```python
from build123d import *

# Parameters (mm, degrees)
F1_DEPTH = 160
F3_DEPTH = 120
F5_DEPTH = 180
F6_R     = 6.35
F7_R     = 6.35


with BuildPart() as f1:
    # F0 (on Front) → F1 (new body)
    with BuildSketch(Plane.XZ):
        with BuildLine():
            Line((140.422905, 79.857803), (-26.877095, 79.857803))
            ThreePointArc((-26.877095, 79.857803), (-31.367223, 77.997931), (-33.227095, 73.507803))
            Line((-33.227095, 73.507803), (-33.227095, -33.792197))
            ThreePointArc((-33.227095, -33.792197), (-31.367223, -38.282325), (-26.877095, -40.142197))
            Line((-26.877095, -40.142197), (140.422905, -40.142197))
            ThreePointArc((140.422905, -40.142197), (144.913033, -38.282325), (146.772905, -33.792197))
            Line((146.772905, -33.792197), (146.772905, 73.507803))
            ThreePointArc((146.772905, 73.507803), (144.913033, 77.997931), (140.422905, 79.857803))
        make_face()
        with BuildLine():
            Line((30.772905, 5.857803), (30.772905, 33.857803))
            ThreePointArc((30.772905, 33.857803), (56.772905, 59.857803), (82.772905, 33.857803))
            Line((82.772905, 33.857803), (82.772905, 5.857803))
            ThreePointArc((82.772905, 5.857803), (56.772905, -20.142197), (30.772905, 5.857803))
        make_face(mode=Mode.SUBTRACT)
    extrude(amount=F1_DEPTH)

    # F2 (on face) → F3 (cut)
    with BuildSketch(Plane(origin=(0, 0, -40.142197), x_dir=(1, 0, 0), z_dir=(0, 0, -1))):
        with BuildLine():
            Line((26.772905, 47.5), (86.772905, 47.5))
            ThreePointArc((86.772905, 47.5), (119.272905, 80), (86.772905, 112.5))
            Line((86.772905, 112.5), (26.772905, 112.5))
            ThreePointArc((26.772905, 112.5), (-5.727095, 80), (26.772905, 47.5))
        make_face()
    extrude(amount=-F3_DEPTH, mode=Mode.SUBTRACT)

    # F4 (on face) → F5 (cut)
    with BuildSketch(Plane(origin=(-33.227095, 0, 0), x_dir=(0, -1, 0), z_dir=(-1, 0, 0))):
        with BuildLine():
            ThreePointArc((108, 31.857803), (80, 59.857803), (52, 31.857803))
            Line((52, 31.857803), (52, 7.857803))
            ThreePointArc((52, 7.857803), (80, -20.142197), (108, 7.857803))
            Line((108, 7.857803), (108, 31.857803))
        make_face()
    extrude(amount=-F5_DEPTH, mode=Mode.SUBTRACT)

    # F6
    f6_edges = [f1.edges().sort_by_distance(p)[0] for p in [
        (56.772905, 0, -40.142197),
        (140.422905, -80, -40.142197),
    ]]
    fillet(f6_edges, radius=F6_R)

    # F7
    f7_edges = [f1.edges().sort_by_distance(p)[0] for p in [
        (56.772905, -160, -40.142197),
        (-26.877095, -83.175, -40.142197),
    ]]
    fillet(f7_edges, radius=F7_R)


solid = f1.part
```
The model under review builds one solid part; all positions refer to its coordinate system, in mm. A direction names the side the tool comes from. Round coordinates to 2 decimals unless told otherwise and drop trailing zeros. Order: outer loops, then holes, each group sorted by start corner. A loop starts at its lowest first (then second) coordinate and runs counter-clockwise, first axis right, second up.
Item 1: Machinability: for faces 1 (the cylindrical face through (56.2, -23.42, 59.85)), 2 (the cylindrical face through (129.55, -80.62, 59.85)), 3 (the flat face through (-33.227, -46, 21)), which of the approach directions +Z, -Z, +X, -X, +Y, -Y give a long, thin tool a straight path to every point of the face, cutting with its end or side? Answer none if there is none.
Working result:
face 1: +Y, -Y
face 2: +X, -X
face 3: +Z, -Z, -X, +Y, -Y
Item 2: Draft analysis for pull direction X (two halves, no side actions). For faces 4 (the cylindrical face through (-31.318, -78.969, 78.047)), 5 (the flat face through (84, -112.5, 19)), 6 (the cylindrical face through (144.86, -158.19, 20.61)), 7 (the cylindrical face through (57.94, -158.19, -38.23)), state which applies: released by +X, released by -X, zero draft, split by the parting line, or undercut.
Working result:
face 4: released by -X
face 5: undercut
face 6: released by +X
face 7: zero draft
Item 3: For pin 1 (6 mm diameter, centred on x = 80, z = 3.5, fed in from +Y), flat-tipped, find the tip position at first contact; note if it passes through.
Working result:
pin 1: stops at y = 0
Item 4: Add section A-A, the plane y = -80. State the section outline as (x, z) points, and give its area (3 significant figures).
Working result:
outline: (-33.23, -33.79) arc R6.35 ccw to (-26.88, -40.14) - (-5.73, -40.14) - (-5.73, -20.14) - (-33.23, -20.14) - close; (-33.23, 59.86) - (-5.73, 59.86) - (-5.73, 79.86) - (-26.88, 79.86) arc R6.35 ccw to (-33.23, 73.51) - close; (119.27, -40.14) - (140.42, -40.14) arc R6.35 ccw to (146.77, -33.79) - (146.77, -20.14) - (119.27, -20.14) - close; (119.27, 59.86) - (146.77, 59.86) - (146.77, 73.51) arc R6.35 ccw to (140.42, 79.86) - (119.27, 79.86) - close
area: 2,170 mm2
Item 5: Add section D-D, the plane x = 57. State the section outline as (y, z) points, and give its area (3 significant figures).
Working result:
outline: (-160, -33.79) arc R6.35 ccw to (-153.65, -40.14) - (-112.5, -40.14) - (-112.5, -20.14) - (-160, -20.14) - close; (-160, 59.86) - (-112.5, 59.86) - (-112.5, 79.86) - (-153.65, 79.86) arc R6.35 ccw to (-160, 73.51) - close; (-47.5, -40.14) - (-6.35, -40.14) arc R6.35 ccw to (0, -33.79) - (0, -20.14) - (-47.5, -20.14) - close; (-47.5, 59.86) - (0, 59.86) - (0, 73.51) arc R6.35 ccw to (-6.35, 79.86) - (-47.5, 79.86) - close
area: 3,770 mm2
Item 6: To check wall thickness, follow probe 1 along Y at (x, z) = (87, 48); probe 2 along Y at (x, z) = (-9.5, 20); probe 3 along X at (y, z) = (-129, 23). State the ranges of each line that lie inside material, in increasing order.
Working result:
probe 1: y = -160 to -112.5, -47.5 to 0
probe 2: y = -160 to -108, -52 to 0
probe 3: x = -33.23 to 30.77, 82.77 to 146.77
Item 7: Add section B-B, the plane x = 91. State the section outline as (y, z) points, and give its area (3 significant figures).
Working result:
outline: (-160, -33.79) arc R6.35 ccw to (-153.65, -40.14) - (-112.22, -40.14) - (-112.22, 79.86) - (-153.65, 79.86) arc R6.35 ccw to (-160, 73.51) - close; (-47.78, -40.14) - (-6.35, -40.14) arc R6.35 ccw to (0, -33.79) - (0, 73.51) arc R6.35 ccw to (-6.35, 79.86) - (-47.78, 79.86) - close
area: 11,400 mm2
Item 8: Add section C-C, the plane z = 69.5. State the section outline as (x, y) points, and give its area (3 significant figures).
Working result:
outline: (-33.23, -153.65) arc R6.35 ccw to (-26.88, -160) - (140.42, -160) arc R6.35 ccw to (146.77, -153.65) - (146.77, -6.35) arc R6.35 ccw to (140.42, 0) - (-26.88, 0) arc R6.35 ccw to (-33.23, -6.35) - close; hole (26.77, -112.5) - (86.77, -112.5) arc R32.5 ccw to (86.77, -47.5) - (26.77, -47.5) arc R32.5 ccw to start
area: 21,500 mm2
